Part model, mm, in its own coordinate system. Coordinates: 2 decimals unless noted, no trailing zeros. Loops run counter-clockwise (first coordinate to the right, second up) from the corner with the lowest first, then second, coordinate; pieces in that order, holes last. Notation, with made-up numbers: (59, -14) - (78, -14) arc R22 cw to (78, 6) - close; hole circle Ø3 at (36.25, 70). An arc over 180 degrees is marked (long way). Use a Markdown table: item, result. Add a question column.
1. Band-saw the part on B-B, the plane x = 48. Give the cut face in (y, z).
2. Drop a flat-ended pin along its axis: pin 1 (12 mm diameter, centred on x = 107.5, z = -15.5, fed in from +Y). Give the stop position or say it passes through.
3. Band-saw the part on A-A, the plane y = 0.6. Count the separate pieces of the cut face and the enclosed holes in it, plus the area to 3 significant figures.
4. Wall check: probe 1 along X at (y, z) = (1.65, -10); probe 2 along Y at (x, z) = (94.5, -12.5); probe 3 along X at (y, z) = (0.4, -32.5). Give the ranges that are in metal, low to high. Write a range as [from, to].
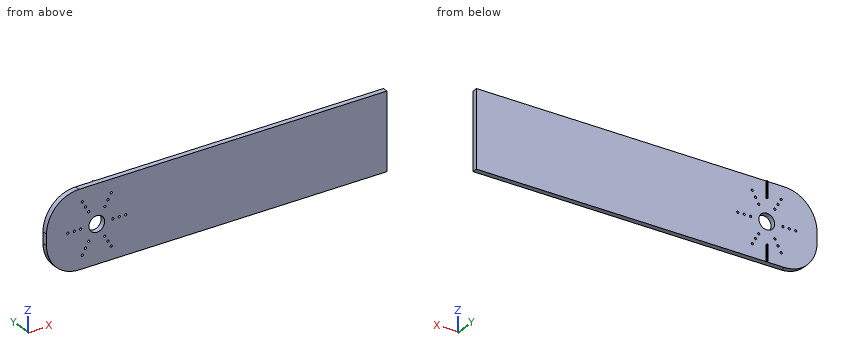
from build123d import *

# Parameters (mm, degrees)
SKETCH1_W           = 157.2
SKETCH1_H           = 35
BOSS_EXTRUDE1_DEPTH = 2.4
SKETCH2_R           = 3.625
SKETCH2_R_2         = 0.5
CUT_EXTRUDE1_DEPTH  = 2.4
SKETCH6_W           = 0.5
SKETCH6_H           = 7.5
BOSS_EXTRUDE3_DEPTH = 0.5
FILLET3_R           = 15


with BuildPart() as part:
    # Sketch1 → Boss-Extrude1 (new body)
    with BuildSketch(Plane(origin=(0, 0, 0), x_dir=(1, 0, 0), z_dir=(0, 1, 0))):
        with Locations((48.922946176, 21.495750708)):
            Rectangle(SKETCH1_W, SKETCH1_H)
    extrude(amount=BOSS_EXTRUDE1_DEPTH)

    # Sketch2 → Cut-Extrude1 (cut)
    with BuildSketch(Plane(origin=(0, 2.4, 0), x_dir=(1, 0, 0), z_dir=(0, 1, 0))):
        with Locations(Location((-6.477053824, 21.495750708, 0), (0, 0, 270))):
            Circle(SKETCH2_R)
        with Locations(Location((-13.907053824, 21.495750708, 0), (0, 0, 270))):
            Circle(SKETCH2_R_2)
        with Locations(Location((-16.842053824, 21.495750708, 0), (0, 0, 270))):
            Circle(SKETCH2_R_2)
        with Locations(Location((-19.847053824, 21.495750708, 0), (0, 0, 270))):
            Circle(SKETCH2_R_2)
        with Locations(Location((-10.192053824, 27.930319458, 0), (0, 0, 270))):
            Circle(SKETCH2_R_2)
        with Locations(Location((-11.659553824, 30.472104018, 0), (0, 0, 270))):
            Circle(SKETCH2_R_2)
        with Locations(Location((-13.162053824, 33.074510357, 0), (0, 0, 270))):
            Circle(SKETCH2_R_2)
        with Locations(Location((-2.762053824, 27.930319458, 0), (0, 0, 270))):
            Circle(SKETCH2_R_2)
        with Locations(Location((-1.294553824, 30.472104018, 0), (0, 0, 270))):
            Circle(SKETCH2_R_2)
        with Locations(Location((0.207946176, 33.074510357, 0), (0, 0, 270))):
            Circle(SKETCH2_R_2)
        with Locations(Location((0.952946176, 21.495750708, 0), (0, 0, 270))):
            Circle(SKETCH2_R_2)
        with Locations(Location((3.887946176, 21.495750708, 0), (0, 0, 270))):
            Circle(SKETCH2_R_2)
        with Locations(Location((6.892946176, 21.495750708, 0), (0, 0, 270))):
            Circle(SKETCH2_R_2)
        with Locations(Location((-2.762053824, 15.061181958, 0), (0, 0, 270))):
            Circle(SKETCH2_R_2)
        with Locations(Location((-1.294553824, 12.519397398, 0), (0, 0, 270))):
            Circle(SKETCH2_R_2)
        with Locations(Location((0.207946176, 9.91699106, 0), (0, 0, 270))):
            Circle(SKETCH2_R_2)
        with Locations(Location((-10.192053824, 15.061181958, 0), (0, 0, 270))):
            Circle(SKETCH2_R_2)
        with Locations(Location((-11.659553824, 12.519397398, 0), (0, 0, 270))):
            Circle(SKETCH2_R_2)
        with Locations(Location((-13.162053824, 9.91699106, 0), (0, 0, 270))):
            Circle(SKETCH2_R_2)
    extrude(amount=-CUT_EXTRUDE1_DEPTH, mode=Mode.SUBTRACT)

    # Sketch6 → Boss-Extrude3 (add)
    with BuildSketch(Plane(origin=(0, 2.4, 0), x_dir=(1, 0, 0), z_dir=(0, 1, 0))):
        with Locations((-6.477053824, 7.745750708)):
            Rectangle(SKETCH6_W, SKETCH6_H)
        with Locations((-6.477053824, 35.245750708)):
            Rectangle(SKETCH6_W, SKETCH6_H)
    extrude(amount=BOSS_EXTRUDE3_DEPTH)

    # Fillet3
    fillet3_edges = [part.edges().sort_by_distance(p)[0] for p in [
        (-29.677053824, 1.2, -38.995750708),
        (-29.677053824, 1.2, -3.995750708),
    ]]
    fillet(fillet3_edges, radius=FILLET3_R)


solid = part.part
Geometry check:
| question | item | result |
|---|---|---|
| 1 | outline | (0, -39) - (2.4, -39) - (2.4, -4) - (0, -4) - close |
| 2 | pin 1 | stops at y = 2.4 |
| 3 | separate pieces | 1 |
| 3 | enclosed holes | 19 |
| 3 | area | 5,350 mm^2 |
| 4 | probe 1 | x = [-26.68, -13.66], [-12.67, -0.29], [0.7, 127.52] |
| 4 | probe 2 | y = [0, 2.4] |
| 4 | probe 3 | x = [-27.03, 127.52] |
